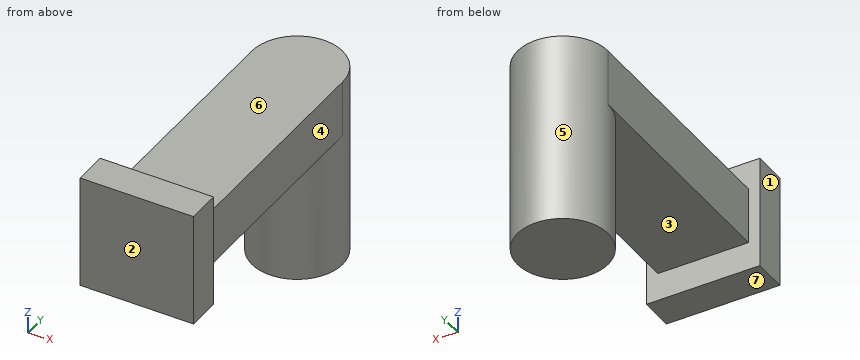
```python
from build123d import *

# Parameters (mm, degrees)
BOSS_EXTRUDE1_START = 13
SKETCH1_R           = 1.9
BOSS_EXTRUDE1_DEPTH = 0.0001
BOSS_EXTRUDE2_START = 13
SKETCH2_R           = 4
BOSS_EXTRUDE2_DEPTH = 17
SKETCH6_W           = 8
SKETCH6_H           = 5
BOSS_EXTRUDE3_DEPTH = 21
SKETCH7_W           = 10
SKETCH7_H           = 10
BOSS_EXTRUDE4_DEPTH = 3


with BuildPart() as part:
    # Sketch1 → Boss-Extrude1 (new body)
    with BuildSketch(Plane.XY.offset(BOSS_EXTRUDE1_START)):
        Circle(SKETCH1_R)
    extrude(amount=BOSS_EXTRUDE1_DEPTH)

    # Sketch2 → Boss-Extrude2 (add)
    with BuildSketch(Plane.XY.offset(BOSS_EXTRUDE2_START)):
        Circle(SKETCH2_R)
    extrude(amount=BOSS_EXTRUDE2_DEPTH)

    # Sketch6 → Boss-Extrude3 (add)
    with BuildSketch(Plane(origin=(0, 0, 0), x_dir=(1, 0, 0), z_dir=(0, 1, 0))):
        with Locations((0, -27.5)):
            Rectangle(SKETCH6_W, SKETCH6_H)
    extrude(amount=-BOSS_EXTRUDE3_DEPTH)

    # Sketch7 → Boss-Extrude4 (add)
    with BuildSketch(Plane.XZ.offset(21)):
        with Locations((0, 27.5)):
            Rectangle(SKETCH7_W, SKETCH7_H)
    extrude(amount=BOSS_EXTRUDE4_DEPTH)


solid = part.part
```
Check sheet for the modelled part. Datum: model origin and axes. Units: mm. Face numbers are marked on the shaded views. A direction names the side the tool comes from. Round coordinates to 2 decimals unless told otherwise and drop trailing zeros. Order: outer loops, then holes, each group sorted by start corner. A loop starts at its lowest first (then second) coordinate and runs counter-clockwise, first axis right, second up. Notation, with made-up numbers: M -25.75,65.25 L -8.75,65.25 A12 cw -8.75,81.25 Z; hole C 18,33 d9. An arc over 180 degrees is marked long. Answer in a Markdown table with one row per item.
(1) Section check C-C on x = 2.25. Record the boundary of the cut face in (y, z).
Findings:
| item | result |
|---|---|
| outline | M -24,22.5 L -21,22.5 L -21,25 L -3.31,25 L -3.31,13 L 3.31,13 L 3.31,30 L -21,30 L -21,32.5 L -24,32.5 Z |
(2) Material ranges on line 1 along Z through (x, y) = (0.5, 2.75); line 2 along X through (y, z) = (-12.5, 27.75); line 3 along Y through (x, z) = (3.5, 31), recorded low to high. Write a range as from..to.
Findings:
| item | result |
|---|---|
| line 1 | z = 13..30 |
| line 2 | x = -4..4 |
| line 3 | y = -24..-21 |
(3) Section check A-A on x = 0. Record the boundary of the cut face in (y, z).
Findings:
| item | result |
|---|---|
| outline | M -24,22.5 L -21,22.5 L -21,25 L -4,25 L -4,13 L 4,13 L 4,30 L -21,30 L -21,32.5 L -24,32.5 Z |
(4) Draft check along Y on the marked faces 1, 2 and 3. Enter one of: +Y half, -Y half, draft (parallel to the pull), parting line (faces both ways), or undercut.
Findings:
| item | result |
|---|---|
| face 1 | draft |
| face 2 | -Y half |
| face 3 | undercut |
(5) Gauge pin test, flat ends, axial feed: pin 1 (2.5 mm diameter, centred on y = -12.5, z = 27.5, fed in from +X); pin 2 (1 mm diameter, centred on x = 0.5, y = -7.5, fed in from +Z); pin 3 (10 mm diameter, centred on y = -20.5, z = 27.5, fed in from -X); pin 4 (1.5 mm diameter, centred on x = -4, y = -9, fed in from -Z). Record the tip position at first contact, or that the pin passes through.
Findings:
| item | result |
|---|---|
| pin 1 | stops at x = 4 |
| pin 2 | stops at z = 30 |
| pin 3 | stops at x = -5 |
| pin 4 | stops at z = 25 |
(6) Section check B-B on y = -12.25. Record the boundary of the cut face in (x, z), plus the area to 3 significant figures.
Findings:
| item | result |
|---|---|
| outline | M -4,25 L 4,25 L 4,30 L -4,30 Z |
| area | 40.0 mm^2 |
(7) Set-up check for the marked faces 4, 5, 6 and 7: record each of +Z, -Z, +X, -X, +Y, -Y from which the full face is reachable in a straight line by a thin tool's end or side.
Findings:
| item | result |
|---|---|
| face 4 | +Z, -Z, +X, +Y |
| face 5 | -Z |
| face 6 | +Z, +X, -X, +Y |
| face 7 | -Z, +X, -X, -Y |
